Could you check a few things on this drawing? It's one solid part, dimensions in mm from its lowest x, y, z. A direction names the side the tool comes from. Give positions to 0.01 mm unless a question says otherwise; leave off trailing zeros. Loops run counter-clockwise (first coordinate to the right, second up) from the corner with the lowest first, then second, coordinate; pieces in that order, holes last. Notation, with made-up numbers: M 23.25,-7.75 L 51.25,-7.75 A26 cw 51.25,13.25 Z; hole C -7.75,-32 d10. An arc over 180 degrees is marked long. One line per item, written item: value. Start each with the question number.
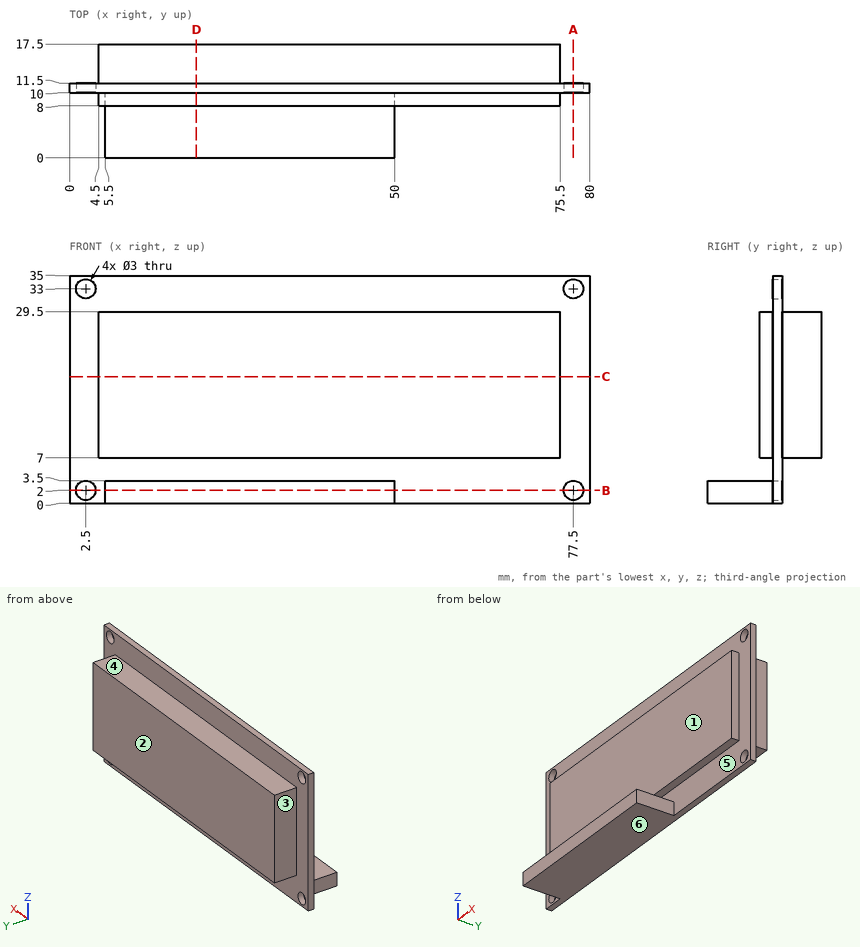
Q1. I need wall thicknesses on line 1 along Z through (x, y) = (77.5, 10.4); line 2 along X through (y, z) = (10.3, 2); line 3 along Z through (x, y) = (20, 13.5). Which ranges of each line are inside material? Lowest first, please.
Q2. If we section it at A-A, the plane x = 77.5: Write out the boundary of the cut face in (y, z), plus the area to 3 significant figures.
Q3. If we section it at C-C, the plane z = 19.5: Write out the boundary of the cut face in (x, y), plus the area to 3 significant figures.
Q4. For P1, Ø3, axis at x = 50.5, y = 13.5, coming from the +Z side; P2, Ø1, axis at y = 3, z = 2.5, coming from the +X side; P3, Ø6.5, axis at y = 15.5, z = 21, coming from the -X side; P4, Ø3, axis at x = 60.5, y = 5, coming from the +Z side, each with a flat end and sliding along its axis, tell me the tip position at first contact or that it passes through.
Q5. If we mould it in two halves opening along Z, with no side actions, what happens to the marked faces 4, 5 and 6? For each: released by +Z, released by -Z, zero draft, split by the parting line, or undercut.
Q6. Which directions (+Z, -Z, +X, -X, +Y, -Y) give clear straight access to the entire face, cutting with the end or side of a thin tool? Please do the marked faces 1, 2 and 3.
Q7. If we section it at B-B, the plane z = 2: Write out the boundary of the cut face in (x, y).
Q8. If we section it at D-D, the plane x = 19.5: Write out the boundary of the cut face in (y, z), plus the area to 4 significant figures.
Response:
1. line 1: 0 to 0.5, 3.5 to 31.5, 34.5 to 35
1. line 2: 0 to 1, 4 to 76, 79 to 80
1. line 3: 7 to 29.5
2. outline: M 10,0 L 11.5,0 L 11.5,0.5 L 10,0.5 Z; M 10,3.5 L 11.5,3.5 L 11.5,31.5 L 10,31.5 Z; M 10,34.5 L 11.5,34.5 L 11.5,35 L 10,35 Z
2. area: 43.5 mm^2
3. outline: M 0,10 L 4.5,10 L 4.5,8 L 75.5,8 L 75.5,10 L 80,10 L 80,11.5 L 75.5,11.5 L 75.5,17.5 L 4.5,17.5 L 4.5,11.5 L 0,11.5 Z
3. area: 688 mm^2
4. P1: z = 29.5
4. P2: x = 50
4. P3: x = 4.5
4. P4: through
5. face 4: released by +Z
5. face 5: undercut
5. face 6: released by -Z
6. face 1: +Z, +X, -X, -Y
6. face 2: +Z, -Z, +X, -X, +Y
6. face 3: +Z, -Z, -X, +Y
7. outline: M 0,10 L 1,10 L 1,11.5 L 0,11.5 Z; M 4,10 L 5.5,10 L 5.5,0 L 50,0 L 50,10 L 76,10 L 76,11.5 L 4,11.5 Z; M 79,10 L 80,10 L 80,11.5 L 79,11.5 Z
8. outline: M 0,0 L 11.5,0 L 11.5,7 L 17.5,7 L 17.5,29.5 L 11.5,29.5 L 11.5,35 L 10,35 L 10,29.5 L 8,29.5 L 8,7 L 10,7 L 10,3.5 L 0,3.5 Z
8. area: 267.5 mm^2
